Autodesk Inventor part; units mm, degrees
ref_plane "YZ Plane" through (0, 0, 0) normal (1, 0, 0) x (0, 1, 0)
ref_plane "XZ Plane" through (0, 0, 0) normal (0, 1, 0) x (-1, 0, 0)
ref_plane "XY Plane" through (0, 0, 0) normal (0, 0, 1) x (1, 0, 0)
sketch "Sketch1" plane through (0, 0, 0) normal (1, 0, 0) x (0, 1, 0)
  line L0 (-12.7, 12.7) -> (12.7, 12.7)
  line L1 (12.7, 12.7) -> (12.7, -12.7)
  line L2 (12.7, -12.7) -> (-12.7, -12.7)
  line L3 (-12.7, -12.7) -> (-12.7, 12.7)
  line L4 (-11.1125, 11.1125) -> (11.1125, 11.1125)
  line L5 (11.1125, 11.1125) -> (11.1125, -10.8514)
  line L6 (11.1125, -10.8514) -> (-11.1125, -10.8514)
  line L7 (-11.1125, -10.8514) -> (-11.1125, 11.1125)
  point P0 (0, 0)
  point P1 (0, 12.7)
  point P2 (-12.7, 0)
  dimension "d0" = 25.4
  dimension "d1" = 25.4
  dimension "d2" = 1.5875
  dimension "d3" = 1.5875
  dimension "d4" = 1.5875
extrude "Extrusion1" add sketch "Sketch1" along normal blind 711.2
sketch "Sketch2" plane through (0, -12.7, 12.7) normal (0, 0, 1) x (1, 0, 0)
  circle A0 centre (9.525, 12.7) radius 6.35
  circle A1 centre (701.675, 12.7) radius 6.35
  line L0 (711.2, 25.4) -> (711.2, 0)
  circle A2 centre (355.6, 12.7) radius 6.35
  line L1 (0, 0) -> (0, 25.4)
  line L2 (0, 0) -> (711.2, 0)
  point P0 (0, 12.7)
  point P1 (393.7, 0)
  point P2 (355.6, 0)
  point P3 (0, 12.7)
  dimension "d7" = 12.7
  dimension "d8" = 9.525
  dimension "d9" = 12.7
  dimension "d10" = 9.525
  dimension "d13" = 12.7
  dimension "d19" = 711.2
extrude "Extrusion4" cut sketch "Sketch2" against normal blind 25.4
equation "\"d1\" = d0"
equation "\"d3\" = d2"
equation "\"d4\" = d2"
equation "\"d9\" = d7"
equation "\"d10\" = d8"
equation "\"d13\" = d7"
properties part number "Long Bar"
Could you check a few things on this model? Use its own coordinates, in mm. A direction names the side the tool comes from. Give positions to 0.01 mm unless a question says otherwise; leave off trailing zeros. Order: outer loops, then holes, each group sorted by start corner. A loop starts at its lowest first (then second) coordinate and runs counter-clockwise, first axis right, second up.
1. I need wall thicknesses on L1, parallel to Z at x = 403.5, y = -5.5; L2, parallel to Y at x = 42.5, z = 4.5; L3, parallel to X at y = 2.75, z = 11.5. Which ranges of each line are inside material? Lowest first, please.
2. We'd pull the mould along X, two halves only. Please class faces 3 (the flat face through (0, -11.3, 0.1)), 4 (the flat face through (351, 11.112, 0)), 5 (the cylindrical face through (361.466, -2.432, 11.917)): pulls with the +X half, pulls with the -X half, needs draft (parallel to the pull), parting line crosses it, or undercut.
3. Suppose I cut it at C-C (y = 0). Give the number of separate pieces and of enclosed holes in the cut face, plus the area to 3 significant figures.
4. Suppose I cut it at B-B (z = -0.75). List the corners of the cut face in (x, y) for me.
5. For faces 1 (the flat face through (351, -11.112, 0)), 2 (the flat face through (351, -5, -12.7)), which set-ups out of +Z, -Z, +X, -X, +Y, -Y let a thin tool reach every point of the face, with its end or its side?
6. Suppose I cut it at A-A (x = 355.6). List the corners of the cut face in (y, z) for me, plus the area to 3 significant figures.
7. Will this pin go through, and if not, where does the flat tip stop? P1, Ø14.5, axis at x = 701.675, y = 0, coming from the +Z side.
Solved:
1. L1: z = -12.7 to -10.85, 11.11 to 12.7
1. L2: y = -12.7 to -11.11, 11.11 to 12.7
1. L3: x = 0 to 3.8, 15.25 to 349.88, 361.32 to 695.95, 707.4 to 711.2
2. face 3: pulls with the -X half
2. face 4: needs draft
2. face 5: undercut
3. separate pieces: 8
3. enclosed holes: 0
3. area: 2,310 mm2
4. outline: (0, -12.7) - (711.2, -12.7) - (711.2, -11.11) - (0, -11.11) - close; (0, 11.11) - (711.2, 11.11) - (711.2, 12.7) - (0, 12.7) - close
5. face 1: +X, -X
5. face 2: -Z, +X, -X, +Y, -Y
6. outline: (-12.7, -12.7) - (-6.35, -12.7) - (-6.35, -10.85) - (-11.11, -10.85) - (-11.11, 11.11) - (-6.35, 11.11) - (-6.35, 12.7) - (-12.7, 12.7) - close; (6.35, -12.7) - (12.7, -12.7) - (12.7, 12.7) - (6.35, 12.7) - (6.35, 11.11) - (11.11, 11.11) - (11.11, -10.85) - (6.35, -10.85) - close
6. area: 113 mm2
7. P1: stops at z = 12.7
